```python
from build123d import *

# Parameters (mm, degrees)
F1_DEPTH = 25.4
F2_DEPTH = 4.7752
F4_D     = 4.7625


# Not quite as in the source:
# - a pattern or mirror of a feature is missing from the dataset's text; its kind, count and spacing are read off the source's solid


with BuildPart() as f1:
    # F0 (on Front) → F1 (new body)
    with BuildSketch(Plane.XZ):
        with BuildLine():
            Line((-35.56, 0), (0, 0))
            Line((0, 0), (35.56, 0))
            Line((35.56, 0), (35.56, 2.54))
            Line((35.56, 2.54), (25.4, 2.54))
            ThreePointArc((25.4, 2.54), (18.6648079092, 5.3298079092), (15.875, 12.065))
            Line((15.875, 12.065), (15.875, 17.526))
            ThreePointArc((15.875, 17.526), (14.351, 19.05), (12.827, 17.526))
            Line((12.827, 17.526), (12.827, 14.097))
            ThreePointArc((12.827, 14.097), (9.0700586823, 5.0269413177), (0, 1.27))
            ThreePointArc((0, 1.27), (-9.0700586823, 5.0269413177), (-12.827, 14.097))
            Line((-12.827, 14.097), (-12.827, 17.526))
            ThreePointArc((-12.827, 17.526), (-14.351, 19.05), (-15.875, 17.526))
            Line((-15.875, 17.526), (-15.875, 12.065))
            ThreePointArc((-15.875, 12.065), (-18.6648079092, 5.3298079092), (-25.4, 2.54))
            Line((-25.4, 2.54), (-35.56, 2.54))
            Line((-35.56, 2.54), (-35.56, 0))
        make_face()
    extrude(amount=F1_DEPTH)

    # F0 (on Front) → F2 (join)
    with BuildSketch(Plane.XZ):
        with BuildLine():
            Line((-35.56, 0), (0, 0))
            Line((0, 0), (35.56, 0))
            Line((35.56, 0), (35.56, 2.54))
            Line((35.56, 2.54), (25.4, 2.54))
            ThreePointArc((25.4, 2.54), (18.6648079092, 5.3298079092), (15.875, 12.065))
            Line((15.875, 12.065), (15.875, 17.526))
            ThreePointArc((15.875, 17.526), (14.351, 19.05), (12.827, 17.526))
            Line((12.827, 17.526), (12.827, 14.097))
            ThreePointArc((12.827, 14.097), (9.0700586823, 5.0269413177), (0, 1.27))
            ThreePointArc((0, 1.27), (-9.0700586823, 5.0269413177), (-12.827, 14.097))
            Line((-12.827, 14.097), (-12.827, 17.526))
            ThreePointArc((-12.827, 17.526), (-14.351, 19.05), (-15.875, 17.526))
            Line((-15.875, 17.526), (-15.875, 12.065))
            ThreePointArc((-15.875, 12.065), (-18.6648079092, 5.3298079092), (-25.4, 2.54))
            Line((-25.4, 2.54), (-35.56, 2.54))
            Line((-35.56, 2.54), (-35.56, 0))
        make_face()
        with BuildLine():
            ThreePointArc((0, 4.699), (-9.0700586823, 8.4559413177), (-12.827, 17.526))
            Line((-12.827, 17.526), (-12.827, 14.097))
            ThreePointArc((-12.827, 14.097), (-9.0700586823, 5.0269413177), (0, 1.27))
            ThreePointArc((0, 1.27), (9.0700586823, 5.0269413177), (12.827, 14.097))
            Line((12.827, 14.097), (12.827, 17.526))
            ThreePointArc((12.827, 17.526), (9.0700586823, 8.4559413177), (0, 4.699))
        make_face()
    extrude(amount=-F2_DEPTH)

    # F4 (through all)
    with Locations(Plane.XY.offset(2.54)):
        with Locations((-30.48, -10.3124)):
            f4 = Hole(F4_D / 2)

    # F4_copies: F4 across plane
    add(f4.mirror(Plane(origin=(0, 0, 0), x_dir=(0, 0, 1), z_dir=(1, 0, 0))), mode=Mode.SUBTRACT)


solid = f1.part
```
Geometry check sheet. Reference: the model listing, model coordinates, mm. A direction names the side the tool comes from. Coordinates: 2 decimals unless noted, no trailing zeros. Loops run counter-clockwise (first coordinate to the right, second up) from the corner with the lowest first, then second, coordinate; pieces in that order, holes last. Notation, with made-up numbers: (-3.75, 84) -> (30.25, 84) arc R7 ccw to (30.25, 96) -> close; hole circle Ø11 at (-18.75, 83.5). An arc over 180 degrees is marked (long way). Put each result on its own line as item: value.
1) Thickness scan on line 1 (Y direction, x = 30.48, z = 1.5); line 2 (X direction, y = -17, z = 15) (3 decimals); line 3 (Z direction, x = -27, y = -14.5). Record the ranges inside material, lowest first.
Result set:
line 1: y = -25.4 to -12.69, -7.93 to 4.78
line 2: x = -15.875 to -12.827, 12.827 to 15.875
line 3: z = 0 to 2.54
2) Tool access check on faces 1 (the flat face through (-15.875, -11, 15)), 2 (the flat face through (0, -11, 0)), 3 (the cylindrical face through (-28.1, -10.2, 1.3)), 4 (the flat face through (15.875, -11, 15)), 5 (the flat face through (12.827, -13, 16)). Record the directions out of +Z, -Z, +X, -X, +Y, -Y that give a thin tool (end or side, any length) a straight path to the whole face; none if there is none.
Result set:
face 1: +Z, -X, +Y, -Y
face 2: -Z, +X, -X, +Y, -Y
face 3: +Z, -Z
face 4: +Z, +X, +Y, -Y
face 5: +Z, -Y
3) Cross-section at C-C on y = -15. Record the boundary of the cut face in (x, z) (3 decimals), plus the area to 3 significant figures.
Result set:
outline: (-35.56, 0) -> (35.56, 0) -> (35.56, 2.54) -> (25.4, 2.54) arc R9.525 cw to (15.875, 12.065) -> (15.875, 17.526) arc R1.524 ccw to (12.827, 17.526) -> (12.827, 14.097) arc R12.827 cw to (-12.827, 14.097) -> (-12.827, 17.526) arc R1.524 ccw to (-15.875, 17.526) -> (-15.875, 12.065) arc R9.525 cw to (-25.4, 2.54) -> (-35.56, 2.54) -> close
area: 356 mm^2
4) Cross-section at B-B on z = 7. Record the boundary of the cut face in (x, y).
Result set:
outline: (-17.33, -25.4) -> (-10.68, -25.4) -> (-10.68, 0) -> (-7.33, 0) -> (-7.33, 4.78) -> (-17.33, 4.78) -> close; (7.33, 0) -> (10.68, 0) -> (10.68, -25.4) -> (17.33, -25.4) -> (17.33, 4.78) -> (7.33, 4.78) -> close
5) Release check for a two-part mould opening along Y. For faces 6 (the cylindrical face through (28.1, -10.2, 1.3)), 7 (the flat face through (0, -25.4, 1)), 8 (the cylindrical face through (-18.591, -10.524, 5.404)) record: released by +Y, released by -Y, zero draft, split by the parting line, or undercut.
Result set:
face 6: undercut
face 7: released by -Y
face 8: zero draft
6) Cross-section at A-A on x = -30.48. Record the boundary of the cut face in (y, z).
Result set:
outline: (-25.4, 0) -> (-12.69, 0) -> (-12.69, 2.54) -> (-25.4, 2.54) -> close; (-7.93, 0) -> (4.78, 0) -> (4.78, 2.54) -> (-7.93, 2.54) -> close
7) Cross-section at D-D on z = 13. Record the boundary of the cut face in (x, y) (3 decimals).
Result set:
outline: (-15.875, -25.4) -> (-12.78, -25.4) -> (-12.78, 0) -> (-12.002, 0) -> (-12.002, 4.775) -> (-15.875, 4.775) -> close; (12.002, 0) -> (12.78, 0) -> (12.78, -25.4) -> (15.875, -25.4) -> (15.875, 4.775) -> (12.002, 4.775) -> close
8) Gauge pin test, flat ends, axial feed: pin 1 Ø1.5 at (x, y) = (0.5, -10) entering from -Z; pin 2 Ø4 at (y, z) = (-15.5, 15.5) entering from -X (3 decimals); pin 3 Ø1 at (y, z) = (-14.5, 16) entering from +X (3 decimals); pin 4 Ø12 at (x, y) = (23.5, -3.5) entering from +Z. Record the tip position at first contact, or that the pin passes through.
Result set:
pin 1: stops at z = 0
pin 2: stops at x = -15.875
pin 3: stops at x = 15.875
pin 4: stops at z = 6.74
